Geometry: final body of the model. Coordinates: model frame, mm. Give positions to 0.01 mm unless a question says otherwise; leave off trailing zeros. Write each loop counter-clockwise with the first axis right and the second up, starting at its lowest first coordinate (ties: lowest second). Pieces come first, ordered by that corner, then holes.
Q1. Pin query (flat end, axial travel): pin 1 Ø4.5 at (x, z) = (-19, 0) entering from -Y; pin 2 Ø8 at (x, z) = (16, -2.5) entering from +Y; pin 3 Ø1 at (y, z) = (44.5, -7) entering from +X; pin 4 Ø2 at (x, y) = (9.5, 32) entering from -Z. Return the tip coordinate at first contact, or that it passes through.
Q2. Mould query, pull axis X, two halves, no side actions, for faces 1 (the flat face through (15, 10, 0)), 2 (the cylindrical face through (-21.747, 4.93, 0.121)), 3 (the cylindrical face through (13.242, 5.063, 19.884)), 4 (the cylindrical face through (12.932, 29.727, -5.362)). Classes: +X half, -X half, draft (parallel to the pull), parting line (faces both ways), or undercut.
Q3. Section D-D (y = 31.5). Return the cut outline in (x, z), plus the area to 3 significant figures.
Q4. Section B-B (z = 0). Return the cut outline in (x, y).
Q5. Section A-A (x = 0). Return the cut outline in (y, z), plus the area to 3 significant figures.
Q6. Line query: line 1 (Z direction, x = 11, y = 9); line 2 (Z direction, x = 0, y = 29); line 3 (Y direction, x = -16, z = 10). Output: solid intervals per line, ascending.
Q7. Section C-C (y = 8.5). Return the cut outline in (x, z), plus the area to 3 significant figures.
from build123d import *

# Parameters (mm, degrees)
F1_R     = 14
F1_R_2   = 8
F2_DEPTH = 50
F1_R_3   = 2.75
F3_DEPTH = 10
F4_R     = 2.5
F5_R     = 0.5


with BuildPart() as f2:
    # F1 (on Front) → F2 (new body)
    with BuildSketch(Plane.XZ):
        Circle(F1_R)
        Circle(F1_R_2, mode=Mode.SUBTRACT)
    extrude(amount=-F2_DEPTH)

    # F1 (on Front) → F3 (join)
    with BuildSketch(Plane.XZ):
        with BuildLine():
            Line((13.266499, 20), (-13.266499, 20))
            ThreePointArc((-13.266499, 20), (-24, 0), (-13.266499, -20))
            Line((-13.266499, -20), (13.266499, -20))
            ThreePointArc((13.266499, -20), (24, 0), (13.266499, 20))
        make_face()
        with Locations((-13.435029, -13.435029)):
            Circle(F1_R_3, mode=Mode.SUBTRACT)
        with Locations((-19, 0)):
            Circle(F1_R_3, mode=Mode.SUBTRACT)
        with Locations((13.435029, -13.435029)):
            Circle(F1_R_3, mode=Mode.SUBTRACT)
        Circle(F1_R, mode=Mode.SUBTRACT)
        with Locations((19, 0)):
            Circle(F1_R_3, mode=Mode.SUBTRACT)
        with Locations((-13.435029, 13.435029)):
            Circle(F1_R_3, mode=Mode.SUBTRACT)
        with Locations((13.435029, 13.435029)):
            Circle(F1_R_3, mode=Mode.SUBTRACT)
    extrude(amount=-F3_DEPTH)

    # F4
    f4_edges = [f2.edges().sort_by_distance(p)[0] for p in [
        (-13.266499, 5, 20),
        (-13.266499, 5, -20),
        (13.266499, 5, 20),
        (13.266499, 5, -20),
    ]]
    fillet(f4_edges, radius=F4_R)

    # F5
    f5_edges = [f2.edges().sort_by_distance(p)[0] for p in [
        (24, 10, 0),
        (24, 0, 0),
        (-14, 10, 0),
        (-14, 50, 0),
    ]]
    fillet(f5_edges, radius=F5_R)


solid = f2.part
Computed:
1. pin 1: passes through
1. pin 2: stops at y = 50
1. pin 3: stops at x = 12.4
1. pin 4: stops at z = -11.12
2. face 1: draft
2. face 2: undercut
2. face 3: +X half
2. face 4: parting line
3. outline: circle Ø28 at (0, 0); hole circle Ø16 at (0, 0)
3. area: 415 mm2
4. outline: (-24, 0.5) arc R0.5 ccw to (-23.5, 0) - (-21.75, 0) - (-21.75, 10) - (-23.5, 10) arc R0.5 ccw to (-24, 9.5) - close; (-16.25, 0) - (-8, 0) - (-8, 50) - (-13.5, 50) arc R0.5 ccw to (-14, 49.5) - (-14, 10.5) arc R0.5 cw to (-14.5, 10) - (-16.25, 10) - close; (8, 0) - (16.25, 0) - (16.25, 10) - (14.5, 10) arc R0.5 cw to (14, 10.5) - (14, 49.5) arc R0.5 ccw to (13.5, 50) - (8, 50) - close; (21.75, 0) - (23.5, 0) arc R0.5 ccw to (24, 0.5) - (24, 9.5) arc R0.5 ccw to (23.5, 10) - (21.75, 10) - close
5. outline: (0, -19.5) arc R0.5 ccw to (0.5, -20) - (9.5, -20) arc R0.5 ccw to (10, -19.5) - (10, -14.5) arc R0.5 cw to (10.5, -14) - (49.5, -14) arc R0.5 ccw to (50, -13.5) - (50, -8) - (0, -8) - close; (0, 8) - (50, 8) - (50, 13.5) arc R0.5 ccw to (49.5, 14) - (10.5, 14) arc R0.5 cw to (10, 14.5) - (10, 19.5) arc R0.5 ccw to (9.5, 20) - (0.5, 20) arc R0.5 ccw to (0, 19.5) - close
5. area: 720 mm2
6. line 1: z = -20 to -14.71, -12.16 to 12.16, 14.71 to 20
6. line 2: z = -14 to -8, 8 to 14
6. line 3: y = 0 to 10
7. outline: (-13.94, -19.53) arc R2.5 ccw to (-12.49, -20) - (12.49, -20) arc R2.5 ccw to (13.94, -19.53) arc R24 ccw to (13.94, 19.53) arc R2.5 ccw to (12.49, 20) - (-12.49, 20) arc R2.5 ccw to (-13.94, 19.53) arc R24 ccw to start; hole circle Ø5.5 at (-19, 0); hole circle Ø5.5 at (-13.44, -13.44); hole circle Ø5.5 at (-13.44, 13.44); hole circle Ø16 at (0, 0); hole circle Ø5.5 at (13.44, -13.44); hole circle Ø5.5 at (13.44, 13.44); hole circle Ø5.5 at (19, 0)
7. area: 1,320 mm2
